```python
from build123d import *

# Parameters (mm, degrees)
SKETCH1_W                  = 480
SKETCH1_H                  = 70
SKETCH1_R                  = 11
SKETCH1_R_2                = 7.1
BOSS_EXTRUDE1_DEPTH        = 10
M5_TAPPED_HOLE1_D          = 4.2
M5_TAPPED_HOLE1_DEPTH      = 10
M5_TAPPED_HOLE1_TIP        = 1.2618073
M5_TAPPED_HOLE2_D          = 4.2
M5_TAPPED_HOLE2_DEPTH      = 12.4
M5_TAPPED_HOLE2_TIP        = 1.2618073
F_3_3_3_3_DIAMETER_HOLE1_D = 3.3


with BuildPart() as part:
    # Sketch1 → Boss-Extrude1 (new body)
    with BuildSketch(Plane.XY):
        Rectangle(SKETCH1_W, SKETCH1_H)
        with Locations((0, -1)):
            Circle(SKETCH1_R, mode=Mode.SUBTRACT)
        with Locations((-215, -5)):
            Circle(SKETCH1_R_2, mode=Mode.SUBTRACT)
        with Locations((215, -5)):
            Circle(SKETCH1_R_2, mode=Mode.SUBTRACT)
    extrude(amount=BOSS_EXTRUDE1_DEPTH)

    # M5 Tapped Hole1
    with Locations(Plane(origin=(0, 35, 0), x_dir=(1, 0, 0), z_dir=(0, 1, 0))):
        with Locations((220, -5), (-220, -5), (-20, -5), (20, -5)):
            Hole(M5_TAPPED_HOLE1_D / 2, depth=M5_TAPPED_HOLE1_DEPTH)
            with Locations((0, 0, -(M5_TAPPED_HOLE1_DEPTH + M5_TAPPED_HOLE1_TIP / 2))):  # 118° drill point
                Cone(0, M5_TAPPED_HOLE1_D / 2, M5_TAPPED_HOLE1_TIP, mode=Mode.SUBTRACT)

    # M5 Tapped Hole2
    with Locations(Plane(origin=(0, -35, 0), x_dir=(-1, 0, 0), z_dir=(0, -1, 0))):
        with Locations((-220, -5), (220, -5)):
            Hole(M5_TAPPED_HOLE2_D / 2, depth=M5_TAPPED_HOLE2_DEPTH)
            with Locations((0, 0, -(M5_TAPPED_HOLE2_DEPTH + M5_TAPPED_HOLE2_TIP / 2))):  # 118° drill point
                Cone(0, M5_TAPPED_HOLE2_D / 2, M5_TAPPED_HOLE2_TIP, mode=Mode.SUBTRACT)

    # Ø3.3 (3.3) Diameter Hole1 (through all)
    with Locations(Plane.XY.offset(10)):
        with Locations((-200, 23), (-120, 23), (-40, 23), (40, 23), (120, 23), (200, 23)):
            Hole(F_3_3_3_3_DIAMETER_HOLE1_D / 2)


solid = part.part
```
Source: CAD feature listing. Evaluate the final solid. Frame: model axes, mm. Give positions to 0.01 mm unless a question says otherwise; leave off trailing zeros. Order: outer loops, then holes, each group sorted by start corner. A loop starts at its lowest first (then second) coordinate and runs counter-clockwise, first axis right, second up. Notation, with made-up numbers: (61.5, 54.25) -> (98.5, 54.25) arc R10 cw to (98.5, 69.25) -> close; hole circle Ø10 at (12.5, 85.5). An arc over 180 degrees is marked (long way). Use a Markdown table: item, result.
Q1. First-contact query: P1, Ø10, axis at x = -116.5, y = -12.5, coming from the -Z side; P2, Ø3, axis at x = -40, y = 23, coming from the +Z side; P3, Ø3.5, axis at x = 220, z = 5, coming from the +Y side; P4, Ø2.5, axis at x = -220, z = 5, coming from the +Y side. Flat tips, straight axial feed; report the tip coordinate or a pass-through.
A:
| item | result |
|---|---|
| P1 | z = 0 |
| P2 | through |
| P3 | y = 24.79 |
| P4 | y = 24.49 |
Q2. Pull-direction query (Y, two-part tool) for faces 1 (the face through (-3, 35, 5)), 2 (the face through (-208.228, -2.867, 4.93)), 3 (the face through (-3, 16, 0)), 4 (the face through (-11, -1, 5)); classes: +Y half, -Y half, draft (parallel to the pull), parting line (faces both ways), or undercut.
A:
| item | result |
|---|---|
| face 1 | +Y half |
| face 2 | undercut |
| face 3 | draft |
| face 4 | undercut |
Q3. Material intervals for line 1 (Y direction, x = -120, z = 3.75); line 2 (Z direction, x = -20, y = 31.75); line 3 (X direction, y = -4.5, z = 8.5), sorted ascending. Write a range as [from, to].
A:
| item | result |
|---|---|
| line 1 | [-35, 21.35], [24.65, 35] |
| line 2 | [0, 2.9], [7.1, 10] |
| line 3 | [-240, -222.08], [-207.92, -10.43], [10.43, 207.92], [222.08, 240] |
Q4. Section A-A (y = -5). Return the cut outline in (x, z), and give its area (3 significant figures).
A:
| item | result |
|---|---|
| outline | (-240, 0) -> (-222.1, 0) -> (-222.1, 10) -> (-240, 10) -> close; (-207.9, 0) -> (-10.25, 0) -> (-10.25, 10) -> (-207.9, 10) -> close; (10.25, 0) -> (207.9, 0) -> (207.9, 10) -> (10.25, 10) -> close; (222.1, 0) -> (240, 0) -> (240, 10) -> (222.1, 10) -> close |
| area | 4,310 mm^2 |
